Geometry: final body of the model. Coordinates: model frame, mm. A direction names the side the tool comes from. Coordinates: 2 decimals unless noted, no trailing zeros. Order: outer loops, then holes, each group sorted by start corner. A loop starts at its lowest first (then second) coordinate and runs counter-clockwise, first axis right, second up. Notation, with made-up numbers: (1, -27.5) -> (6, -27.5) arc R32 ccw to (6, 3.5) -> close; hole circle Ø6 at (79, 58.5). An arc over 180 degrees is marked (long way). Answer in a Markdown table with one row per item. Add a question column.
1) Section query A-A on y = 22.5. Count the separate pieces of the cut face and the enclosed holes in it, then the cut area to 3 significant figures.
2) Ray query, line 1 (X direction, y = 31.5, z = 0); line 2 (X direction, y = 28, z = -21); line 3 (Z direction, x = -3.5, y = 20.5). Return the intervals inside material, ascending. Write a range as from..to.
3) Contact query for flat-ended pins moving along their axis: P1, Ø5, axis at x = -4.13, z = -0.19, coming from the +Y side; P2, Ø5, axis at x = 2.5, y = 17.5, coming from the -Z side; P3, Ø2, axis at x = -4.5, z = 20, coming from the +Y side; P4, Ø1.8, axis at x = -29.13, z = -25.19, coming from the +Y side. Output: stop coordinate, or through.
4) Section query B-B on x = -11. Return the cut outline in (y, z).
5) Pull-direction query (X, two-part tool) for faces 4 (the face through (17, 4.9, 28)), 5 (the face through (-24, 16, -30.193)), 6 (the face through (25.874, 16, -24)); classes: +X half, -X half, draft (parallel to the pull), parting line (faces both ways), or undercut.
6) Set-up query: faces 1 (the face through (-1.026, 19.096, -11.169)), 2 (the face through (-5.604, 2.416, 0.42)), 3 (the face through (6, 17, -17.193)). Return all of +Z, -Z, +X, -X, +Y, -Y with unobstructed straight access to the full face (end or side cutting, diameter ignored); none if empty.
```python
from build123d import *

# Parameters (mm, degrees)
SKETCH1_W                      = 80
SKETCH1_H                      = 80
BOSS_EXTRUDE1_DEPTH            = 32.9
M2_5X0_45_TAPPED_HOLE1_D       = 2.05
M2_5X0_45_TAPPED_HOLE1_DEPTH   = 6.35
M2_5X0_45_TAPPED_HOLE1_TIP     = 0.615882135
CBORE_FOR_M3_SHCS1_D           = 3.2
CBORE_FOR_M3_SHCS1_CBORE_D     = 6.5
CBORE_FOR_M3_SHCS1_CBORE_DEPTH = 28
SKETCH25_W                     = 40
SKETCH25_H                     = 32.9
CUT_EXTRUDE2_DEPTH             = 13


with BuildPart() as part:
    # Sketch1 → Boss-Extrude1 (new body)
    with BuildSketch(Plane(origin=(0, 0, 0), x_dir=(1, 0, 0), z_dir=(0, 1, 0))):
        with Locations((5.874226931, -9.806779272)):
            Rectangle(SKETCH1_W, SKETCH1_H)
    extrude(amount=BOSS_EXTRUDE1_DEPTH)

    # M2.5x0.45 Tapped Hole1
    with Locations(Plane(origin=(-29.125773069, 32.9, -25.193220728), x_dir=(0, 0, 1), z_dir=(0, 1, 0))):
        with Locations((0, 0), (0, 70), (70, 70), (70, 0)):
            Hole(M2_5X0_45_TAPPED_HOLE1_D / 2, depth=M2_5X0_45_TAPPED_HOLE1_DEPTH)
            with Locations((0, 0, -(M2_5X0_45_TAPPED_HOLE1_DEPTH + M2_5X0_45_TAPPED_HOLE1_TIP / 2))):  # 118° drill point
                Cone(0, M2_5X0_45_TAPPED_HOLE1_D / 2, M2_5X0_45_TAPPED_HOLE1_TIP, mode=Mode.SUBTRACT)

    # CBORE for M3 SHCS1 (through all)
    with Locations(Plane(origin=(0, 32.9, 0), x_dir=(1, 0, 0), z_dir=(0, 1, 0))):
        with Locations((15.874226931, -29.806779272), (-4.125773069, -29.806779272), (-4.125773069, -19.806779272), (-4.125773069, -9.806779272), (-4.125773069, 0.193220728), (-4.125773069, 10.193220728), (15.874226931, -19.806779272), (15.874226931, -9.806779272), (15.874226931, 0.193220728), (15.874226931, 10.193220728)):
            CounterBoreHole(CBORE_FOR_M3_SHCS1_D / 2, CBORE_FOR_M3_SHCS1_CBORE_D / 2, CBORE_FOR_M3_SHCS1_CBORE_DEPTH)

    # Sketch25 → Cut-Extrude2 (cut)
    with BuildSketch(Plane(origin=(0, 0, -30.193220728), x_dir=(-1, 0, 0), z_dir=(0, 0, -1))):
        with Locations((-5.874226931, 16.45)):
            Rectangle(SKETCH25_W, SKETCH25_H)
    extrude(amount=-CUT_EXTRUDE2_DEPTH, mode=Mode.SUBTRACT)


solid = part.part
```
Result:
| question | item | result |
|---|---|---|
| 1 | separate pieces | 1 |
| 1 | enclosed holes | 10 |
| 1 | area | 5,550 mm2 |
| 2 | line 1 | -34.13..-7.37, -0.88..12.63, 19.12..45.87 |
| 2 | line 2 | -34.13..-14.13, 25.87..45.87 |
| 2 | line 3 | -17.19..-13.38, -7..-3.38, 3..6.62, 13..16.62, 23..26.62, 33..49.81 |
| 3 | P1 | y = 4.9 |
| 3 | P2 | z = -17.19 |
| 3 | P3 | through |
| 3 | P4 | y = 26.48 |
| 4 | outline | (0, -17.19) -> (32.9, -17.19) -> (32.9, 49.81) -> (0, 49.81) -> close |
| 5 | face 4 | undercut |
| 5 | face 5 | draft |
| 5 | face 6 | undercut |
| 6 | face 1 | +Y |
| 6 | face 2 | +Y, -Y |
| 6 | face 3 | -Z, +Y, -Y |
